Could you check a few things on this drawing? It's one solid part, dimensions in mm from its lowest x, y, z. Give positions to 0.01 mm unless a question says otherwise; leave off trailing zeros. Order: outer loops, then holes, each group sorted by start corner. A loop starts at its lowest first (then second) coordinate and runs counter-clockwise, first axis right, second up.
Item 1: If I drill on line 1 along Y through (x, z) = (10.5, 28.5) (1 decimal); line 2 along Y through (x, z) = (13.75, 86.5) (1 decimal); line 3 along Z through (x, y) = (20, 81.5), over which ranges is the centre line in solid material (lowest first)?
Item 2: I want a section at B-B, the plane z = 44. Write out the boundary of the cut face in (x, y), then the cut area to 3 significant figures.
Item 3: If we mould it in two halves opening along Y, with no side actions, what happens to the marked faces 1, 2 and 3? For each: +Y half, -Y half, draft (parallel to the pull), parting line (faces both ways), or undercut.
Item 4: I'm going to push flat-ended pins straight in: pin 1 Ø8 at (x, z) = (5, 103) entering from -Y (1 decimal); pin 2 Ø5 at (x, z) = (6, 69) entering from -Y; pin 3 Ø2 at (x, y) = (3.5, 113) entering from -Z; pin 4 Ø3 at (y, z) = (78, 105) entering from -X. Where does each tip first touch, or does it pass through?
Item 5: I want a section at C-C, the plane y = 118. Write out the boundary of the cut face in (x, z) (1 decimal), then the cut area to 3 significant figures.
Item 6: I want a section at A-A, the plane x = 19.25. Write out the boundary of the cut face in (y, z), then the cut area to 3 significant figures.
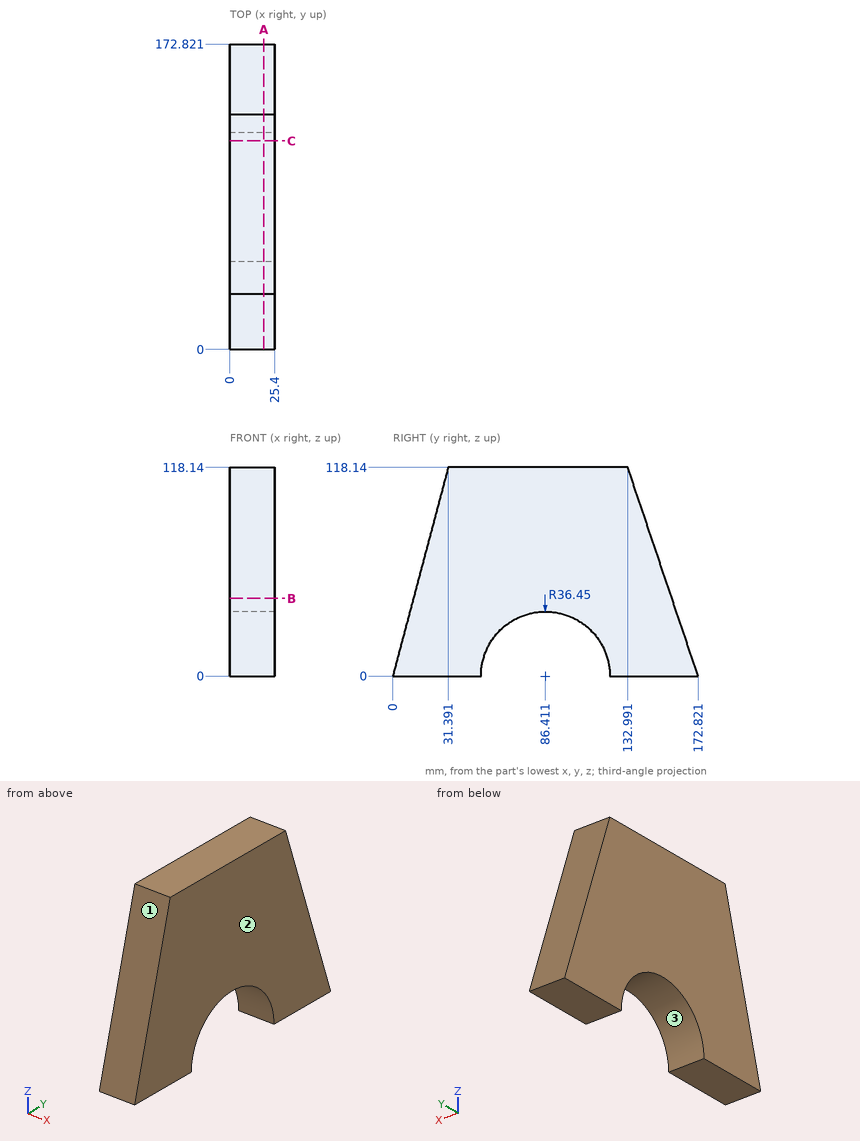
Results list:
1. line 1: y = 7.6 to 63.7, 109.1 to 163.2
1. line 2: y = 23 to 143.7
1. line 3: z = 36.12 to 118.14
2. outline: (0, 11.69) - (25.4, 11.69) - (25.4, 157.99) - (0, 157.99) - close
2. area: 3,720 mm2
3. face 1: -Y half
3. face 2: draft
3. face 3: undercut
4. pin 1: stops at y = 26.3
4. pin 2: stops at y = 17.67
4. pin 3: stops at z = 23.82
4. pin 4: stops at x = 0
5. outline: (0, 18.2) - (25.4, 18.2) - (25.4, 118.1) - (0, 118.1) - close
5. area: 2,540 mm2
6. outline: (0, 0) - (49.96, 0) arc R36.45 cw to (122.86, 0) - (172.82, 0) - (132.99, 118.14) - (31.39, 118.14) - close
6. area: 14,100 mm2
